The listing builds one solid part. Answer for the finished solid, in the listing's coordinates (mm). Face numbers are marked on the shaded views. A direction names the side the tool comes from. Round coordinates to 2 decimals unless told otherwise and drop trailing zeros. Write each loop counter-clockwise with the first axis right and the second up, starting at its lowest first coordinate (ties: lowest second). Pieces come first, ordered by that corner, then holes. Notation, with made-up numbers: (58.25, -9.5) - (101.25, -9.5) arc R23 ccw to (101.25, 25.5) - close; hole circle Ø7 at (30.25, 26.25). An arc over 180 degrees is marked (long way). Use a Markdown table: item, result. Add a question column.
1) A cutting plane is placed at B-B (x = -24). Give the vertices of the cut face in (y, z), then the cut area to 3 significant figures.
2) A cutting plane is placed at C-C (z = -7.5). Give the vertices of the cut face in (x, y), then the cut area to 3 significant figures.
3) A cutting plane is placed at A-A (y = 1.5). Give the vertices of the cut face in (x, z), then the cut area to 3 significant figures.
4) A tool of negligible diameter and unlimited length cuts with its end or side. For the marked faces 1 and 2, from which of +Z, -Z, +X, -X, +Y, -Y can it reach the whole face along a straight path? Write none if from no direction.
5) Determine the mould class of the marked faces 3, 4, 5 and 6 for opening direction Z: +Z half, -Z half, draft (parallel to the pull), parting line (faces both ways), or undercut.
6) Find the intervals of material crossed by probe 1 along Z at (x, y) = (8.5, 4); probe 2 along Y at (x, z) = (2.5, 26); probe 3 along Z at (x, y) = (-3, -25), in increasing order. Write a range as from..to.
7) A cutting plane is placed at D-D (y = -12). Give the vertices of the cut face in (x, z), then the cut area to 3 significant figures.
8) Each of these flat-tipped pins is pushed along its axis until it touches: P1, Ø1.5, axis at x = -22, y = -21.5, coming from the +Z side; P2, Ø1.5, axis at x = -32.5, z = 27, coming from the +Y side. Where does it stop, or does it pass through?
```python
from build123d import *

# Parameters (mm, degrees)
SKETCH1_W           = 90
SKETCH1_H           = 57
BOSS_EXTRUDE1_DEPTH = 60
FILLET1_R           = 20
SHELL1_T            = -2
FILLET2_R           = 10


with BuildPart() as part:
    # Sketch1 → Boss-Extrude1 (new, symmetric)
    with BuildSketch(Plane.XY):
        Rectangle(SKETCH1_W, SKETCH1_H)
    extrude(amount=BOSS_EXTRUDE1_DEPTH, both=True)

    # Fillet1
    fillet1_edges = [part.edges().sort_by_distance(p)[0] for p in [
        (0, -28.5, 60),
        (0, -28.5, -60),
    ]]
    fillet(fillet1_edges, radius=FILLET1_R)

    # Shell1
    shell1_openings = [part.faces().sort_by_distance(p)[0] for p in [
        (-45, 0.618740562, 0),
        (0, 28.5, 0),
        (45, 0.618740562, 0),
    ]]
    offset(amount=SHELL1_T, openings=shell1_openings, kind=Kind.INTERSECTION)

    # Fillet2
    fillet2_edges = [part.edges().sort_by_distance(p)[0] for p in [
        (-45, 28.5, -59),
        (45, 28.5, -59),
        (-45, 28.5, 59),
        (45, 28.5, 59),
    ]]
    fillet(fillet2_edges, radius=FILLET2_R)


solid = part.part
```
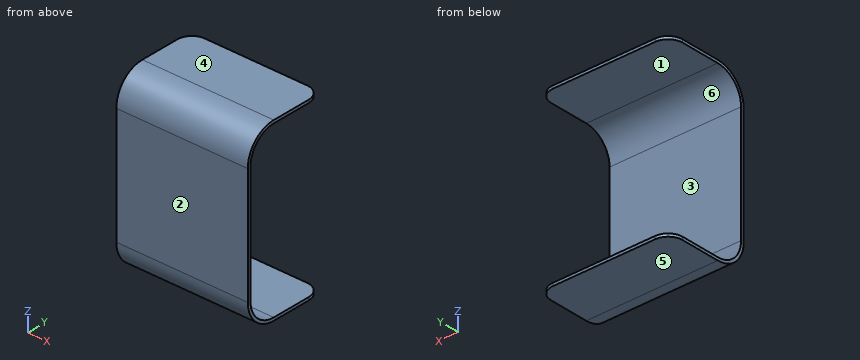
Entries:
| question | item | result |
|---|---|---|
| 1 | outline | (-28.5, -40) arc R20 ccw to (-8.5, -60) - (28.5, -60) - (28.5, -58) - (-8.5, -58) arc R18 cw to (-26.5, -40) - (-26.5, 40) arc R18 cw to (-8.5, 58) - (28.5, 58) - (28.5, 60) - (-8.5, 60) arc R20 ccw to (-28.5, 40) - close |
| 1 | area | 427 mm² |
| 2 | outline | (-45, -28.5) - (45, -28.5) - (45, -26.5) - (-45, -26.5) - close |
| 2 | area | 180 mm² |
| 3 | outline | (-45, -60) - (45, -60) - (45, -58) - (-45, -58) - close; (-45, 58) - (45, 58) - (45, 60) - (-45, 60) - close |
| 3 | area | 360 mm² |
| 4 | face 1 | +X, -X, +Y |
| 4 | face 2 | +Z, -Z, +X, -X, -Y |
| 5 | face 3 | undercut |
| 5 | face 4 | +Z half |
| 5 | face 5 | -Z half |
| 5 | face 6 | undercut |
| 6 | probe 1 | z = -60..-58, 58..60 |
| 6 | probe 2 | y = -28.5..-26.5 |
| 6 | probe 3 | z = -51.3..-47.19, 47.19..51.3 |
| 7 | outline | (-45, -59.69) - (45, -59.69) - (45, -57.66) - (-45, -57.66) - close; (-45, 57.66) - (45, 57.66) - (45, 59.69) - (-45, 59.69) - close |
| 7 | area | 366 mm² |
| 8 | P1 | stops at z = 55.81 |
| 8 | P2 | stops at y = -26.5 |
